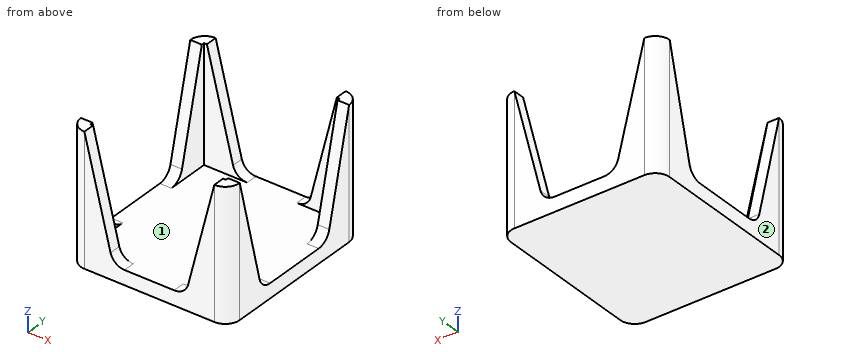
from build123d import *

# Parameters (mm, degrees)
F0_W         = 55
F0_H         = 60
F1_DEPTH     = 5
F3_DEPTH     = 40
F5_T4_DEPTH  = 211.7701999818
F5_T9_DEPTH  = 211.7701999818
F5_T14_DEPTH = 211.7701999818
F5_T19_DEPTH = 211.7701999818
F5_T24_DEPTH = 211.7701999818
F5_T29_DEPTH = 211.7701999818
F5_T34_DEPTH = 211.7701999818
F5_T39_DEPTH = 211.7701999818
F7_R         = 5
F8_R         = 5


# Not quite as in the source:
# - a fillet or chamfer that OpenCascade refuses, or shapes differently, is made with other operations: its cross-section is extruded or revolved along the edge and cut away or added
# - two fillets or chamfers of one size are made in one step
# - a feature of the source that left no trace in its solid (it failed there, or was rolled back) is left out


with BuildPart() as f1:
    # F0 (on Top) → F1 (new body)
    with BuildSketch(Plane.XY):
        Rectangle(F0_W, F0_H)
    extrude(amount=F1_DEPTH)

    # F2 (on face) → F3 (join)
    with BuildSketch(Plane.XY.offset(5)):
        Polygon((-23.5, 15), (-23.5, 26), (-12.5, 26), (-12.5, 30), (-27.5, 30), (-27.5, 15), align=None)
        Polygon((12.5, 30), (12.5, 26), (23.5, 26), (23.5, 15), (27.5, 15), (27.5, 30), align=None)
        Polygon((23.5, -26), (12.5, -26), (12.5, -30), (27.5, -30), (27.5, -15), (23.5, -15), align=None)
        Polygon((-23.5, -26), (-23.5, -15), (-27.5, -15), (-27.5, -30), (-12.5, -30), (-12.5, -26), align=None)
    extrude(amount=F3_DEPTH)

    # F5: chamfer of 10 x 40 on 8 edges, made by hand


with BuildPart() as f5_tool2:
    # F5_s3 → F5_t4 (new body)
    with BuildSketch(Plane.YZ.offset(-131.3850999909)):
        Polygon((15, 5), (25, 45), (15, 45), align=None)
    extrude(amount=F5_T4_DEPTH)

    split(bisect_by=Plane.XY.offset(5), keep=Keep.TOP)


with BuildPart() as f1_1:
    add(f1.part)

    # F5_t1: cut F5_tool2
    add(f5_tool2.part, mode=Mode.SUBTRACT)


with BuildPart() as f5_tool7:
    # F5_s8 → F5_t9 (new body)
    with BuildSketch(Plane.XZ.offset(-77.8850999909)):
        Polygon((22.5, 45), (12.5, 5), (12.5, 45), align=None)
    extrude(amount=F5_T9_DEPTH)

    split(bisect_by=Plane.XY.offset(5), keep=Keep.TOP)


with BuildPart() as f1_2:
    add(f1_1.part)

    # F5_t6: cut F5_tool7
    add(f5_tool7.part, mode=Mode.SUBTRACT)


with BuildPart() as f5_tool12:
    # F5_s13 → F5_t14 (new body)
    with BuildSketch(Plane.YZ.offset(-80.3850999909)):
        Polygon((15, 5), (25, 45), (15, 45), align=None)
    extrude(amount=F5_T14_DEPTH)

    split(bisect_by=Plane.XY.offset(5), keep=Keep.TOP)


with BuildPart() as f1_3:
    add(f1_2.part)

    # F5_t11: cut F5_tool12
    add(f5_tool12.part, mode=Mode.SUBTRACT)


with BuildPart() as f5_tool17:
    # F5_s18 → F5_t19 (new body)
    with BuildSketch(Plane.XZ.offset(-133.8850999909)):
        Polygon((12.5, 5), (22.5, 45), (12.5, 45), align=None)
    extrude(amount=F5_T19_DEPTH)

    split(bisect_by=Plane.XY.offset(5), keep=Keep.TOP)


with BuildPart() as f1_4:
    add(f1_3.part)

    # F5_t16: cut F5_tool17
    add(f5_tool17.part, mode=Mode.SUBTRACT)


with BuildPart() as f5_tool22:
    # F5_s23 → F5_t24 (new body)
    with BuildSketch(Plane.YZ.offset(131.3850999909)):
        Polygon((-25, 45), (-15, 5), (-15, 45), align=None)
    extrude(amount=-F5_T24_DEPTH)

    split(bisect_by=Plane.XY.offset(5), keep=Keep.TOP)


with BuildPart() as f1_5:
    add(f1_4.part)

    # F5_t21: cut F5_tool22
    add(f5_tool22.part, mode=Mode.SUBTRACT)


with BuildPart() as f5_tool27:
    # F5_s28 → F5_t29 (new body)
    with BuildSketch(Plane.XZ.offset(133.8850999909)):
        Polygon((-12.5, 5), (-22.5, 45), (-12.5, 45), align=None)
    extrude(amount=-F5_T29_DEPTH)

    split(bisect_by=Plane.XY.offset(5), keep=Keep.TOP)


with BuildPart() as f1_6:
    add(f1_5.part)

    # F5_t26: cut F5_tool27
    add(f5_tool27.part, mode=Mode.SUBTRACT)


with BuildPart() as f5_tool32:
    # F5_s33 → F5_t34 (new body)
    with BuildSketch(Plane.YZ.offset(80.3850999909)):
        Polygon((-15, 5), (-25, 45), (-15, 45), align=None)
    extrude(amount=-F5_T34_DEPTH)

    split(bisect_by=Plane.XY.offset(5), keep=Keep.TOP)


with BuildPart() as f1_7:
    add(f1_6.part)

    # F5_t31: cut F5_tool32
    add(f5_tool32.part, mode=Mode.SUBTRACT)


with BuildPart() as f5_tool37:
    # F5_s38 → F5_t39 (new body)
    with BuildSketch(Plane.XZ.offset(77.8850999909)):
        Polygon((-22.5, 45), (-12.5, 5), (-12.5, 45), align=None)
    extrude(amount=-F5_T39_DEPTH)

    split(bisect_by=Plane.XY.offset(5), keep=Keep.TOP)


with BuildPart() as f1_8:
    add(f1_7.part)

    # F5_t36: cut F5_tool37
    add(f5_tool37.part, mode=Mode.SUBTRACT)

    # F7
    f7_edges = [f1_8.edges().sort_by_distance(p)[0] for p in [
        (-27.5, -30, 22.5),
        (27.5, -30, 22.5),
        (27.5, 30, 22.5),
        (-27.5, 30, 22.5),
    ]]
    fillet(f7_edges, radius=F7_R)

    # F8
    f8_edges = [f1_8.edges().sort_by_distance(p)[0] for p in [
        (12.5, -28, 5),
        (12.5, 28, 5),
        (25.5, 15, 5),
        (-25.5, 15, 5),
        (-12.5, 28, 5),
        (-25.5, -15, 5),
        (-12.5, -28, 5),
        (25.5, -15, 5),
    ]]
    fillet(f8_edges, radius=F8_R)


solid = f1_8.part
For this review, take the finished solid that the model builds, in its own axes (mm). Face numbers are marked on the shaded views. A direction names the side the tool comes from. Round coordinates to 2 decimals unless told otherwise and drop trailing zeros. Write each loop counter-clockwise with the first axis right and the second up, starting at its lowest first coordinate (ties: lowest second). Pieces come first, ordered by that corner, then holes. Notation, with made-up numbers: (-8, 28.25) - (18, 28.25) arc R32 cw to (18, 57.25) - close; hole circle Ø1 at (72, 85). An arc over 180 degrees is marked (long way). Write item = value, one per line. Start each with the question number.
1. Consider section C-C on y = -18. State the section outline as (x, z) points, plus the area to 3 significant figures.
2. For pin 1 Ø16.5 at (y, z) = (-20.5, 29) entering from +X; pin 2 Ø16.5 at (x, y) = (-6, 1) entering from +Z, all flat-tipped, find the tip position at first contact; note any pin that passes through.
3. Wall thickness on L1, parallel to Y at x = -20.5, z = 16; L2, parallel to Z at x = 20, y = -6; L3, parallel to X at y = 21.5, z = 8.5: over which ranges is each line inside the solid? List them lowest first.
4. For the marked faces 1 and 2, list the 3-axis set-ups (+Z, -Z, +X, -X, +Y, -Y) from which the entire face can be reached by the end or side of a thin tool; tool diameter is ignored.
5. Consider section D-D on z = 29. State the section outline as (x, y) points, plus the area to 3 significant figures.
6. Consider section A-A on z = 21. State the section outline as (x, y) points.
7. Consider section B-B on x = -17. State the section outline as (y, z) points.
Evaluation:
q1.outline = (-27.5, 0) - (27.5, 0) - (27.5, 17) - (23.5, 17) - (23.5, 5) - (-23.5, 5) - (-23.5, 17) - (-27.5, 17) - close
q1.area = 371 mm2
q2.pin_1 = 27.5
q2.pin_2 = 5
q3.L1 = -30 to -26, 26 to 30
q3.L2 = 0 to 5
q3.L3 = -27.5 to -23.5, 23.5 to 27.5
q4.face_1 = +Z
q4.face_2 = +Z, -Z, -X, +Y, -Y
q5.outline = (-27.5, -25) arc R5 ccw to (-22.5, -30) - (-18.5, -30) - (-18.5, -26) - (-23.5, -26) - (-23.5, -21) - (-27.5, -21) - close; (-27.5, 21) - (-23.5, 21) - (-23.5, 26) - (-18.5, 26) - (-18.5, 30) - (-22.5, 30) arc R5 ccw to (-27.5, 25) - close; (18.5, -30) - (22.5, -30) arc R5 ccw to (27.5, -25) - (27.5, -21) - (23.5, -21) - (23.5, -26) - (18.5, -26) - close; (18.5, 26) - (23.5, 26) - (23.5, 21) - (27.5, 21) - (27.5, 25) arc R5 ccw to (22.5, 30) - (18.5, 30) - close
q5.area = 203 mm2
q6.outline = (-27.5, -25) arc R5 ccw to (-22.5, -30) - (-16.5, -30) - (-16.5, -26) - (-23.5, -26) - (-23.5, -19) - (-27.5, -19) - close; (-27.5, 19) - (-23.5, 19) - (-23.5, 26) - (-16.5, 26) - (-16.5, 30) - (-22.5, 30) arc R5 ccw to (-27.5, 25) - close; (16.5, -30) - (22.5, -30) arc R5 ccw to (27.5, -25) - (27.5, -19) - (23.5, -19) - (23.5, -26) - (16.5, -26) - close; (16.5, 26) - (23.5, 26) - (23.5, 19) - (27.5, 19) - (27.5, 25) arc R5 ccw to (22.5, 30) - (16.5, 30) - close
q7.outline = (-30, 0) - (30, 0) - (30, 23) - (26, 23) - (26, 5) - (-26, 5) - (-26, 23) - (-30, 23) - close
